Could you check a few things on this drawing? It's one solid part, dimensions in mm from its lowest x, y, z. Give positions to 0.01 mm unless a question says otherwise; leave off trailing zeros. Order: outer loops, then holes, each group sorted by start corner. A loop starts at its lowest first (then second) coordinate and runs counter-clockwise, first axis right, second up.
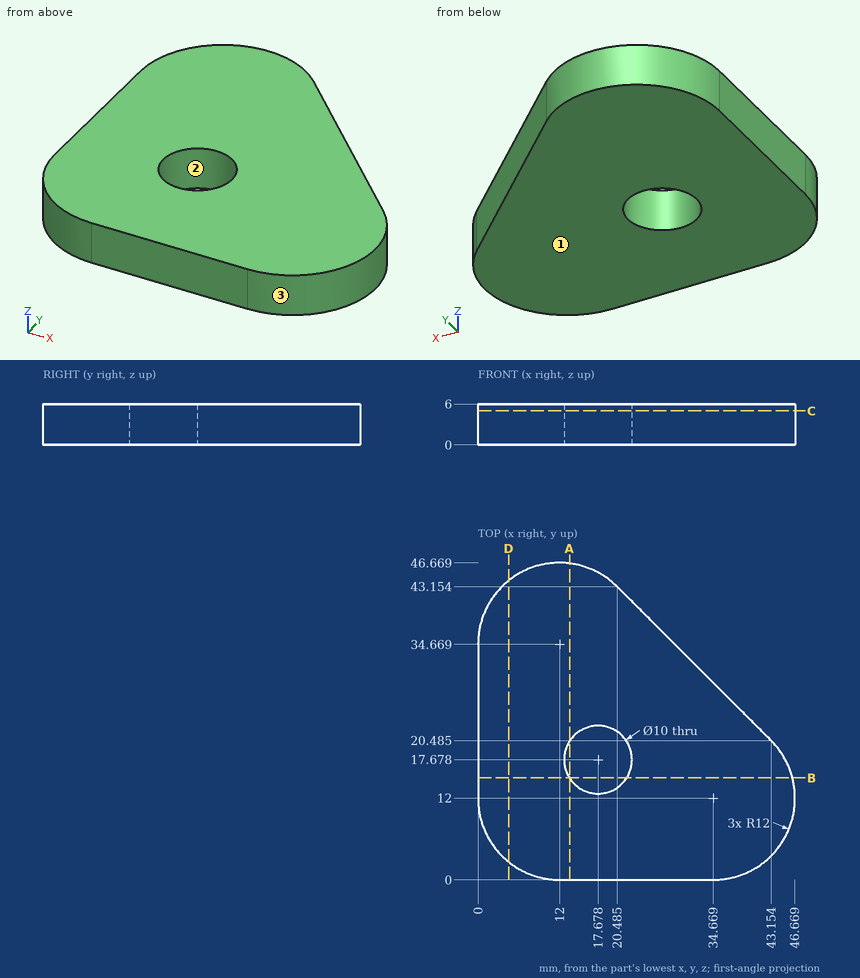
1) We'd pull the mould along X, two halves only. Please class the marked faces 1, 2 and 3: +X half, -X half, draft (parallel to the pull), parting line (faces both ways), or undercut.
2) Suppose I cut it at C-C (z = 5). Please give me the cut outline in (x, y) (1 decimal), and give its area (3 significant figures).
3) If I drill on line 1 (X direction, y = 14, z = 2.5) (1 decimal); line 2 (Y direction, x = 17.5, z = 3.7) (1 decimal); line 3 (X direction, y = 16, z = 5.4), over which ranges is the centre line in solid material (lowest first)?
4) Suppose I cut it at B-B (y = 15). Please give me the cut outline in (x, z) (1 decimal).
5) Suppose I cut it at A-A (x = 13.5). Please give me the cut outline in (y, z) (1 decimal).
6) Suppose I cut it at D-D (x = 4.5). Please give me the cut outline in (y, z).
Results:
1. face 1: draft
1. face 2: undercut
1. face 3: +X half
2. outline: (0, 12) arc R12 ccw to (12, 0) - (34.7, 0) arc R12 ccw to (43.2, 20.5) - (20.5, 43.2) arc R12 ccw to (0, 34.7) - close; hole circle Ø10 at (17.7, 17.7)
2. area: 1,560 mm2
3. line 1: x = 0 to 14.3, 21.1 to 46.5
3. line 2: y = 0 to 12.7, 22.7 to 45.3
3. line 3: x = 0 to 12.97, 22.39 to 45.98
4. outline: (0, 0) - (13.5, 0) - (13.5, 6) - (0, 6) - close; (21.9, 0) - (46.3, 0) - (46.3, 6) - (21.9, 6) - close
5. outline: (0, 0) - (14.9, 0) - (14.9, 6) - (0, 6) - close; (20.4, 0) - (46.6, 0) - (46.6, 6) - (20.4, 6) - close
6. outline: (2.63, 0) - (44.04, 0) - (44.04, 6) - (2.63, 6) - close
